Geometry check sheet. Reference: the model listing, model coordinates, mm. A direction names the side the tool comes from. Coordinates: 2 decimals unless noted, no trailing zeros. Loops run counter-clockwise (first coordinate to the right, second up) from the corner with the lowest first, then second, coordinate; pieces in that order, holes last. Notation, with made-up numbers: (-3, 28) -> (9, 28) arc R7 ccw to (9, 40) -> close; hole circle Ø9 at (7.5, 59.25). An arc over 180 degrees is marked (long way). Answer as a JSON object with one key per item and string values.
from build123d import *

# Parameters (mm, degrees)
F1_DEPTH = 35
F2_W     = 30
F2_H     = 30
F3_DEPTH = 60
F4_R     = 5
F5_DEPTH = 10.001
F7_DEPTH = 70.001
F9_DEPTH = 10


with BuildPart() as f1:
    # F0 (on Front) → F1 (new body, symmetric)
    with BuildSketch(Plane.XZ):
        with BuildLine():
            Line((0, 40), (0, 0))
            Line((0, 0), (70, 0))
            Line((70, 0), (70, 60))
            Line((70, 60), (20, 60))
            ThreePointArc((20, 60), (14.142136, 45.857864), (0, 40))
        make_face()
    extrude(amount=F1_DEPTH, both=True)

    # F2 (on face) → F3 (cut)
    with BuildSketch(Plane.XZ.offset(35)):
        with Locations((55, 45)):
            Rectangle(F2_W, F2_H)
    extrude(amount=-F3_DEPTH, mode=Mode.SUBTRACT)

    # F4 (on face) → F5 (cut, through all)
    with BuildSketch(Plane.XZ.offset(-25)):
        with Locations((55, 45)):
            Circle(F4_R)
    extrude(amount=-F5_DEPTH, mode=Mode.SUBTRACT)

    # F6 (on face) → F7 (cut, through all)
    with BuildSketch(Plane.YZ.offset(70)):
        with BuildLine():
            ThreePointArc((20, 0), (0, 20), (-20, 0))
            Line((-20, 0), (20, 0))
        make_face()
    extrude(amount=-F7_DEPTH, mode=Mode.SUBTRACT)

    # F8 (on face) → F9 (join)
    with BuildSketch(Plane.XZ.offset(35)):
        with BuildLine():
            Line((0, 40), (0, 29.999999))
            ThreePointArc((0, 29.999999), (21.213204, 38.786796), (30.000001, 60))
            Line((30.000001, 60), (20, 60))
            ThreePointArc((20, 60), (14.142136, 45.857864), (0, 40))
        make_face()
    extrude(amount=F9_DEPTH)

    # F10: F1 across plane


with BuildPart() as f1_1:
    add(f1.part)
    add(f1.part.mirror(Plane.YZ))


solid = f1_1.part
1. Mould release check, pull along X, two halves, no side actions. Record for faces 4 (the face through (-70, 0, 23)), 5 (the face through (1, -35, 24)), 6 (the face through (40, -5, 45)), 7 (the face through (-54.349, 29.93, 49.957)): released by +X, released by -X, zero draft, split by the parting line, or undercut.
Evaluation:
{"face 4": "released by -X", "face 5": "zero draft", "face 6": "released by +X", "face 7": "undercut"}
2. Thickness scan on probe 1 along Z at (x, y) = (55, 32.25); probe 2 along Y at (x, z) = (63, 29.5); probe 3 along Z at (x, y) = (-40.5, -25.5). Record the ranges inside material, lowest first. Write a range as from..to.
Evaluation:
{"probe 1": "z = 0..40, 50..60", "probe 2": "y = -35..35", "probe 3": "z = 0..30"}
3. Depth check by flat-ended pin: P1, Ø24, axis at y = -19.5, z = 52, coming from the -X side; P2, Ø2, axis at x = -1.5, y = -34, coming from the +Z side; P3, Ø9, axis at x = 60.5, y = -7.5, coming from the +Z side. Enter the tip coordinate at first touch or a pass-through.
Evaluation:
{"P1": "stops at x = -40", "P2": "stops at z = 40.16", "P3": "stops at z = 30"}
4. Section check B-B, the plane z = 48. Record the boundary of the cut face in (x, y).
Evaluation:
{"outline": "(-70, 25) -> (-59, 25) -> (-59, 35) -> (-70, 35) -> close; (-51, 25) -> (-40, 25) -> (-40, -35) -> (-27.5, -35) -> (-27.5, -45) -> (-16, -45) -> (-16, 35) -> (-51, 35) -> close; (16, -45) -> (27.5, -45) -> (27.5, -35) -> (40, -35) -> (40, 25) -> (51, 25) -> (51, 35) -> (16, 35) -> close; (59, 25) -> (70, 25) -> (70, 35) -> (59, 35) -> close"}
5. Section check A-A, the plane x = -55. Record the boundary of the cut face in (y, z), then the cut area to 3 significant figures.
Evaluation:
{"outline": "(-35, 0) -> (-20, 0) arc R20 cw to (20, 0) -> (35, 0) -> (35, 40) -> (25, 40) -> (25, 30) -> (-35, 30) -> close; (25, 50) -> (35, 50) -> (35, 60) -> (25, 60) -> close", "area": "1,670 mm^2"}
6. Tool access check on faces 1 (the face through (-40, -5, 45)), 2 (the face through (0, -45, 39)), 3 (the face through (51, 25, 49)). Record the directions out of +Z, -Z, +X, -X, +Y, -Y that give a thin tool (end or side, any length) a straight path to the whole face; none if there is none.
Evaluation:
{"face 1": "+Z, -X, -Y", "face 2": "+Z, -Z, +X, -X, -Y", "face 3": "+Z, +X, -Y"}
7. Section check C-C, the plane y = 7. Record the boundary of the cut face in (x, z) (3 decimals), then the cut area to 3 significant figures.
Evaluation:
{"outline": "(-70, 18.735) -> (70, 18.735) -> (70, 30) -> (40, 30) -> (40, 60) -> (20, 60) arc R20 cw to (0, 40) arc R20 cw to (-20, 60) -> (-40, 60) -> (-40, 30) -> (-70, 30) -> close", "area": "3,350 mm^2"}
8. Section check D-D, the plane x = -35. Record the boundary of the cut face in (y, z), then the cut area to 3 significant figures.
Evaluation:
{"outline": "(-35, 0) -> (-20, 0) arc R20 cw to (20, 0) -> (35, 0) -> (35, 60) -> (-35, 60) -> close", "area": "3,570 mm^2"}
